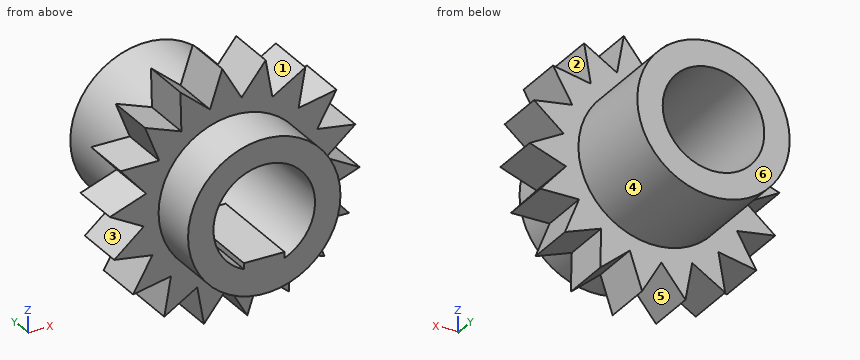
```python
from build123d import *

# Parameters (mm, degrees)
SKETCH1_R           = 9
BOSS_EXTRUDE1_DEPTH = 5
SKETCH2_R           = 7.5
BOSS_EXTRUDE2_DEPTH = 10
SKETCH3_R           = 5
CUT_EXTRUDE1_DEPTH  = 20
SKETCH4_W           = 4
SKETCH4_H           = 2
BOSS_EXTRUDE3_DEPTH = 10


with BuildPart() as part:
    # Sketch1 → Boss-Extrude1 (new body)
    with BuildSketch(Plane(origin=(0, 0, 0), x_dir=(1, 0, 0), z_dir=(0, 1, 0))):
        Circle(SKETCH1_R)
        Polygon((-5.35288104, -11.104144955), (-5.256580304, -7.305365392), (-8.827904062, -8.603689933), (-7.438151841, -5.066941601), (-11.238151569, -5.065502929), (-8.72257249, -2.217369874), (-12.292912138, -0.916341513), (-8.954922165, 0.899649385), (-11.86496608, 3.343344214), (-8.107176067, 3.908157651), (-10.005930004, 7.199773285), (-6.281584886, 6.445284426), (-6.940031098, 10.187803442), (-3.698341861, 8.205014776), (-3.037062017, 11.947034147), (-0.669024226, 8.975099252), (1.232221565, 12.265276214), (2.440987604, 8.6626543), (5.35288104, 11.104144955), (5.256580304, 7.305365392), (8.827904062, 8.603689933), (7.438151841, 5.066941601), (11.238151569, 5.065502929), (8.72257249, 2.217369874), (12.292912138, 0.916341513), (8.954922165, -0.899649385), (11.86496608, -3.343344214), (8.107176067, -3.908157651), (10.005930004, -7.199773285), (6.281584886, -6.445284426), (6.940031098, -10.187803442), (3.698341861, -8.205014776), (3.037062017, -11.947034147), (0.669024226, -8.975099252), (-1.232221565, -12.265276214), (-2.440987604, -8.6626543), align=None)
    extrude(amount=BOSS_EXTRUDE1_DEPTH)

    # Sketch2 → Boss-Extrude2 (add, symmetric)
    with BuildSketch(Plane(origin=(0, 5, 0), x_dir=(1, 0, 0), z_dir=(0, 1, 0))):
        Circle(SKETCH2_R)
    extrude(amount=BOSS_EXTRUDE2_DEPTH, both=True)

    # Sketch3 → Cut-Extrude1 (cut)
    with BuildSketch(Plane(origin=(0, 15, 0), x_dir=(1, 0, 0), z_dir=(0, 1, 0))):
        Circle(SKETCH3_R)
    extrude(amount=-CUT_EXTRUDE1_DEPTH, mode=Mode.SUBTRACT)

    # Sketch4 → Boss-Extrude3 (add)
    with BuildSketch(Plane(origin=(0, 5, 0), x_dir=(1, 0, 0), z_dir=(0, 1, 0))):
        with Locations((0, 5)):
            Rectangle(SKETCH4_W, SKETCH4_H)
    extrude(amount=-BOSS_EXTRUDE3_DEPTH)


solid = part.part
```
Input: part model. Units: mm. Frame: model coordinates. Face numbers are marked on the shaded views. A direction names the side the tool comes from. Give positions to 0.01 mm unless a question says otherwise; leave off trailing zeros. Order: outer loops, then holes, each group sorted by start corner. A loop starts at its lowest first (then second) coordinate and runs counter-clockwise, first axis right, second up. Notation, with made-up numbers: M -6.75,34 L 39.25,34 A15 cw 39.25,40 Z; hole C -27,39.5 d1. An arc over 180 degrees is marked long. Return JSON: item names as keys, results as strings.
1) Access query for the marked faces 1, 2 and 3. Directions: +Z, -Z, +X, -X, +Y, -Y. A direction counts if a zero-diameter tool reaches every point of the face in a straight line with its end or side. Return the directions, or none.
Taken from the geometry:
{"face 1": "+Z, +Y, -Y", "face 2": "+Y, -Y", "face 3": "-X, +Y, -Y"}
2) Contact query for flat-ended pins moving along their axis: pin 1 (3 mm diameter, centred on x = 8.5, z = -8, fed in from -Y); pin 2 (10 mm diameter, centred on y = 1, z = -7, fed in from -X); pin 3 (1.9 mm diameter, centred on x = -9.5, y = 3, fed in from +Z). Output: stop coordinate, or through.
Taken from the geometry:
{"pin 1": "stops at y = 0", "pin 2": "stops at x = -11.86", "pin 3": "stops at z = 8.6"}
3) Section query D-D on x = 10.5. Output: boundary loops of the cut face in (y, z), and give its area (3 significant figures).
Taken from the geometry:
{"outline": "M 0,-5.07 L 5,-5.07 L 5,-4.23 L 0,-4.23 Z; M 0,-1.57 L 5,-1.57 L 5,0.06 L 0,0.06 Z; M 0,2.2 L 5,2.2 L 5,3.55 L 0,3.55 Z", "area": "19.1 mm2"}
4) Mould query, pull axis X, two halves, no side actions, for the marked faces 4, 5 and 6. Classes: released by +X, released by -X, zero draft, split by the parting line, or undercut.
Taken from the geometry:
{"face 4": "split by the parting line", "face 5": "undercut", "face 6": "zero draft"}
5) Section query A-A on x = 4.25. Output: boundary loops of the cut face in (y, z), and give its area (3 significant figures).
Taken from the geometry:
{"outline": "M -5,-6.18 L 0,-6.18 L 0,-10.18 L 5,-10.18 L 5,-6.18 L 15,-6.18 L 15,-2.63 L -5,-2.63 Z; M -5,2.63 L 15,2.63 L 15,6.18 L 5,6.18 L 5,8.54 L 0,8.54 L 0,6.18 L -5,6.18 Z", "area": "174 mm2"}
6) Section query C-C on z = 0. Output: boundary loops of the cut face in (x, y).
Taken from the geometry:
{"outline": "M -10.61,0 L -7.5,0 L -7.5,-5 L -5,-5 L -5,15 L -7.5,15 L -7.5,5 L -10.61,5 Z; M 5,-5 L 7.5,-5 L 7.5,0 L 10.61,0 L 10.61,5 L 7.5,5 L 7.5,15 L 5,15 Z"}
7) Section query B-B on y = -1. Output: boundary loops of the cut face in (x, z).
Taken from the geometry:
{"outline": "C 0,0 d15; hole M -2,-4.58 L -2,-4 L 2,-4 L 2,-4.58 A5 ccw long Z"}
8) Line query: L1, parallel to Z at x = 0, y = 5.75; L2, parallel to X at y = 0.75, z = 0. Output: solid intervals per line, ascending. Write a range as [from, to].
Taken from the geometry:
{"L1": "z = [-7.5, -5], [5, 7.5]", "L2": "x = [-10.61, -5], [5, 10.61]"}
